Check sheet for the drawn part. Datum: minimum x, y, z corner. Units: mm. Round coordinates to 2 decimals unless told otherwise and drop trailing zeros. Write each loop counter-clockwise with the first axis right and the second up, starting at its lowest first coordinate (ties: lowest second). Pieces come first, ordered by that corner, then holes. Notation, with made-up numbers: (-32.75, 23.25) - (-11.75, 23.25) arc R31 ccw to (-11.75, 48.25) - close; hole circle Ø10 at (70.25, -26). An arc over 180 degrees is marked (long way). Write each question's results on one line, items separated by ' | '.
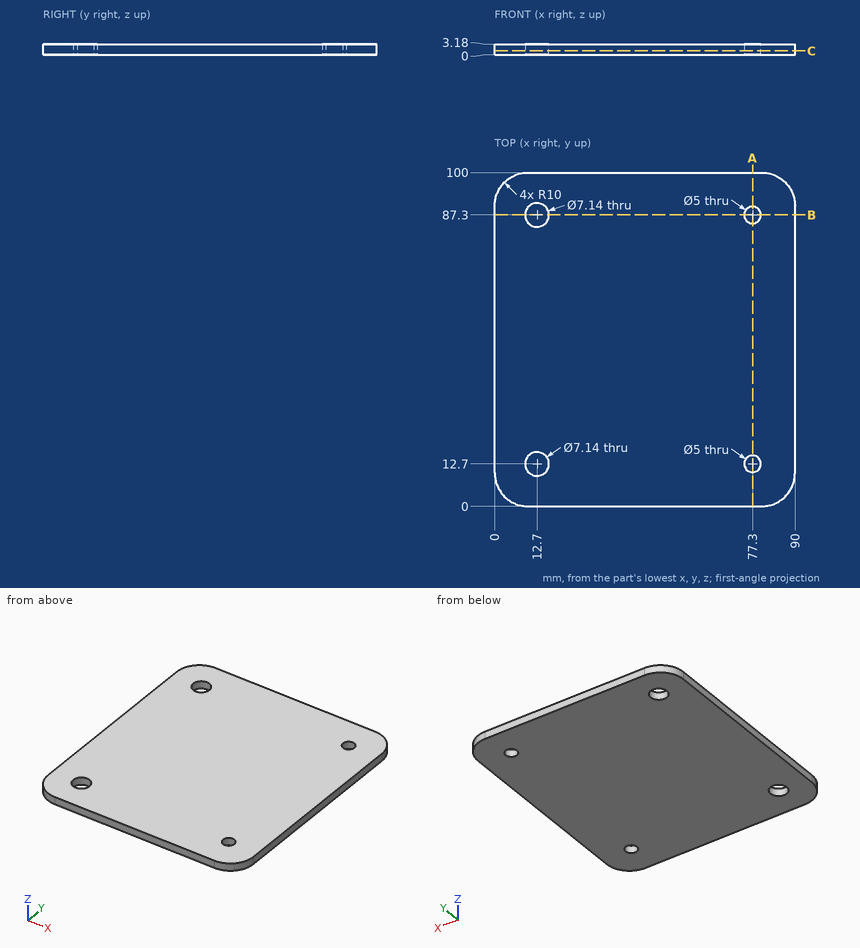
(1) Section check A-A (x = 77.3). Record the cut outline in (y, z).
Answer:
outline: (0, 0) - (10.2, 0) - (10.2, 3.18) - (0, 3.18) - close; (15.2, 0) - (84.8, 0) - (84.8, 3.18) - (15.2, 3.18) - close; (89.8, 0) - (100, 0) - (100, 3.18) - (89.8, 3.18) - close
(2) Section check C-C (z = 1.1). Record the cut outline in (x, y).
Answer:
outline: (0, 10) arc R10 ccw to (10, 0) - (80, 0) arc R10 ccw to (90, 10) - (90, 90) arc R10 ccw to (80, 100) - (10, 100) arc R10 ccw to (0, 90) - close; hole circle Ø7.14 at (12.7, 12.7); hole circle Ø7.14 at (12.7, 87.3); hole circle Ø5 at (77.3, 12.7); hole circle Ø5 at (77.3, 87.3)
(3) Thickness scan on L1, parallel to Y at x = 12.7, z = 1.15; L2, parallel to Y at x = 77.3, z = 1.2; L3, parallel to X at y = 15, z = 2.35. Record the ranges inside material, lowest first.
Answer:
L1: 0 to 9.13, 16.27 to 83.73, 90.87 to 100 | L2: 0 to 10.2, 15.2 to 84.8, 89.8 to 100 | L3: 0 to 9.97, 15.43 to 76.32, 78.28 to 90
(4) Section check B-B (y = 87.3). Record the cut outline in (x, z).
Answer:
outline: (0, 0) - (9.13, 0) - (9.13, 3.18) - (0, 3.18) - close; (16.27, 0) - (74.8, 0) - (74.8, 3.18) - (16.27, 3.18) - close; (79.8, 0) - (90, 0) - (90, 3.18) - (79.8, 3.18) - close
(5) Go/stop test with a flat-tipped pin: pin 1 Ø6.5 at (x, y) = (77.3, 87.3) entering from +Z. Record where the tip stops, or that it passes through.
Answer:
pin 1: z = 3.18
